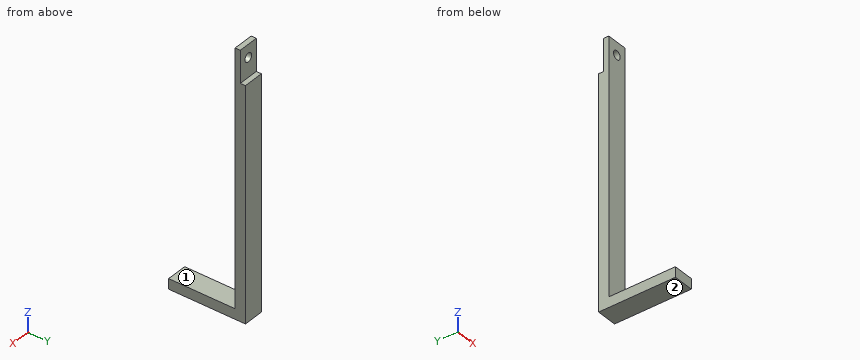
Autodesk Inventor part; units mm, degrees
ref_plane "YZ Plane" through (0, 0, 0) normal (1, 0, 0) x (0, 1, 0)
ref_plane "XZ Plane" through (0, 0, 0) normal (0, 1, 0) x (-1, 0, 0)
ref_plane "XY Plane" through (0, 0, 0) normal (0, 0, 1) x (1, 0, 0)
sketch "Sketch1" plane through (0, 0, 0) normal (0, 1, 0) x (-1, 0, 0)
  line L0 (0, 0) -> (8, 0)
  line L1 (8, 0) -> (8, 98.806)
  line L2 (8, 98.806) -> (0, 98.806)
  line L3 (0, 98.806) -> (0, 0)
  line L4 (4, 0) -> (4, 98.806)
  line L5 (4, 98.806) -> (4, 93.806)
  circle A0 centre (4, 93.806) radius 1.7
  dimension "d0" = 8
  dimension "d1" = 98.806
  dimension "d2" = 90
  dimension "d3" = 8
  dimension "d4" = 98.806
  dimension "d5" = 5
  dimension "d6" = 3.4
extrude "Extrusion1" add sketch "Sketch1" along normal blind 4 contours L3 L2 L4 A0 L0 | L4 A0 L2 L1 L0
sketch "Sketch2" plane through (-8, 0, 98.806) normal (0, 0, 1) x (1, 0, 0)
  line L0 (8, 4) -> (0, 4)
  line L1 (0, 4) -> (8, 4)
  line L2 (8, 4) -> (8, 2)
  line L3 (8, 2) -> (0, 2)
  line L4 (0, 2) -> (0, 4)
  point P0 (8, 0)
  dimension "d9" = 8
  dimension "d10" = 2
extrude "Extrusion2" cut sketch "Sketch2" against normal blind 12.54
sketch "Sketch3" plane through (0, 4, 0) normal (0, 1, 0) x (1, 0, 0)
  line L0 (0, 0) -> (-8, 0)
  line L1 (0, 0) -> (-8, 0)
  line L2 (-8, 0) -> (-8, 4)
  line L3 (-8, 4) -> (0, 4)
  line L4 (0, 4) -> (0, 0)
  dimension "d13" = 8
  dimension "d14" = 4
extrude "Extrusion3" add sketch "Sketch3" against normal blind 30
properties part number "brace1"
Design review of the part built by this model. Coordinates are the model's own, in mm. Face numbers are marked on the shaded views. A direction names the side the tool comes from. Coordinates: 2 decimals unless noted, no trailing zeros. Write each loop counter-clockwise with the first axis right and the second up, starting at its lowest first coordinate (ties: lowest second). Pieces come first, ordered by that corner, then holes. Notation, with made-up numbers: (7, 8.25) - (48, 8.25) arc R9 ccw to (48, 16.25) - close; hole circle Ø3 at (29, -2.75). An arc over 180 degrees is marked (long way). One line per item, written item: value.
1) Insertion check: pin 1 (1 mm diameter, centred on x = -1, z = 87, fed in from -Y); pin 2 (2 mm diameter, centred on x = -4, z = 93.806, fed in from +Y); pin 3 (2 mm diameter, centred on x = -1.5, z = 87.5, fed in from +Y); pin 4 (4 mm diameter, centred on x = -3, y = -6.5, fed in from +Z). Each pin has a flat end and moves straight along its axis. Give the tip position at first contact, or say it passes through.
Answer sheet:
pin 1: stops at y = 0
pin 2: passes through
pin 3: stops at y = 2
pin 4: stops at z = 0
2) Add section C-C (y = -7.5). State the section outline as (x, z) points, plus the area to 3 significant figures.
Answer sheet:
outline: (-8, -4) - (0, -4) - (0, 0) - (-8, 0) - close
area: 32.0 mm2
3) Add section B-B (z = 11.5). State the section outline as (x, y) points.
Answer sheet:
outline: (-8, 0) - (0, 0) - (0, 4) - (-8, 4) - close
4) Add section A-A (x = -4). State the section outline as (y, z) points, plus the area to 3 significant figures.
Answer sheet:
outline: (-26, -4) - (4, -4) - (4, 86.27) - (2, 86.27) - (2, 92.11) - (0, 92.11) - (0, 0) - (-26, 0) - close; (0, 95.51) - (2, 95.51) - (2, 98.81) - (0, 98.81) - close
area: 483 mm2
5) To check wall thickness, follow probe 1 along Z at (x, y) = (-4, 1.1); probe 2 along Y at (x, z) = (-1.5, 77); probe 3 along Z at (x, y) = (-0.5, -9.5). State the ranges of each line that lie inside material, in increasing order.
Answer sheet:
probe 1: z = -4 to 92.11, 95.51 to 98.81
probe 2: y = 0 to 4
probe 3: z = -4 to 0
6) For the marked faces 1 and 2, list the 3-axis set-ups (+Z, -Z, +X, -X, +Y, -Y) from which the entire face can be reached by the end or side of a thin tool; tool diameter is ignored.
Answer sheet:
face 1: +Z, +X, -X, -Y
face 2: -Z, +X, -X, +Y, -Y
